Autodesk Inventor part; units mm, degrees
ref_plane "YZ Plane" through (0, 0, 0) normal (1, 0, 0) x (0, 1, 0)
ref_plane "XZ Plane" through (0, 0, 0) normal (0, 1, 0) x (-1, 0, 0)
ref_plane "XY Plane" through (0, 0, 0) normal (0, 0, 1) x (1, 0, 0)
sketch "Sketch1" plane through (0, 0, 0) normal (0, 1, 0) x (-1, 0, 0)
  line L0 (10.3823, 13.6045) -> (-19.4881, 13.6045)
  line L1 (-19.4881, 13.6045) -> (-19.4881, -34.6555)
  line L2 (-19.4881, -34.6555) -> (10.3823, -34.6555)
  line L3 (10.3823, -34.6555) -> (10.3823, 13.6045)
  point P0 (0, 0)
  dimension "d0" = 48.26
  dimension "d1" = 29.8704
extrude "Extrusion1" add sketch "Sketch1" along normal blind 20.193
fillet "Fillet1" radius 3.175 2 edges at (19.4881, 20.193, -10.5255) (-10.3823, 20.193, -10.5255)
sketch "Sketch2" plane through (0, 0, 0) normal (0, -1, 0) x (1, 0, 0)
  line L0 (13.0111, -34.6555) -> (13.0111, -42.2755)
  line L1 (19.4881, 13.6045) -> (19.4881, -34.6555)
  line L2 (13.0111, -42.2755) -> (6.7881, -42.2755)
  line L3 (6.7881, -42.2755) -> (6.7881, -34.6555)
  line L4 (6.7881, -36.6113) -> (2.3177, -36.6113)
  line L5 (2.3177, -34.6555) -> (2.3177, -42.2755)
  line L6 (2.3177, -42.2755) -> (-3.9053, -42.2755)
  line L7 (-3.9053, -42.2755) -> (-3.9053, -34.6555)
  line L8 (-10.3823, -34.6555) -> (-10.3823, 13.6045)
  line L9 (19.4881, -10.5255) -> (-10.3823, -10.5255) construction
  line L10 (13.0111, 13.6045) -> (13.0111, 21.2245)
  line L11 (13.0111, 21.2245) -> (6.7881, 21.2245)
  line L12 (6.7881, 21.2245) -> (6.7881, 13.6045)
  line L13 (6.7881, 15.5603) -> (2.3177, 15.5603)
  line L14 (2.3177, 13.6045) -> (2.3177, 21.2245)
  line L15 (2.3177, 21.2245) -> (-3.9053, 21.2245)
  line L16 (-3.9053, 21.2245) -> (-3.9053, 13.6045)
  line L17 (13.0111, -34.6555) -> (6.7881, -34.6555)
  line L18 (2.3177, -34.6555) -> (-3.9053, -34.6555)
  line L19 (19.4881, -34.6555) -> (-10.3823, -34.6555)
  line L20 (6.7881, -34.6555) -> (2.3177, -34.6555)
  line L21 (13.0111, 13.6045) -> (6.7881, 13.6045)
  line L22 (-10.3823, 13.6045) -> (19.4881, 13.6045)
  line L23 (6.7881, 13.6045) -> (2.3177, 13.6045)
  line L24 (2.1667, 13.6045) -> (-3.9053, 13.6045)
  line L25 (6.7881, 13.6045) -> (2.3177, 13.6045)
  line L26 (2.3177, 13.6045) -> (2.3177, 15.5603)
  line L27 (2.3177, 15.5603) -> (6.7881, 15.5603)
  line L28 (6.7881, 15.5603) -> (6.7881, 13.6045)
  line L29 (6.7881, -36.6113) -> (2.3177, -36.6113)
  line L30 (2.3177, -36.6113) -> (2.3177, -34.6555)
  line L31 (2.3177, -34.6555) -> (6.7881, -34.6555)
  line L32 (6.7881, -34.6555) -> (6.7881, -36.6113)
  line L33 (-3.9053, 13.6045) -> (2.3177, 13.6045)
  line L34 (2.3177, 13.6045) -> (2.3177, 21.2245)
  line L35 (2.3177, 21.2245) -> (-3.9053, 21.2245)
  line L36 (-3.9053, 21.2245) -> (-3.9053, 13.6045)
  point P0 (0, 0)
  dimension "d5" = 6.477
  dimension "d6" = 7.62
  dimension "d7" = 6.223
  dimension "d9" = 4.4704
  dimension "d10" = 6.223
  dimension "d11" = 7.62
  dimension "d12" = 29.8704
  dimension "d13" = 4.4704
  dimension "d15" = 6.477
  dimension "d16" = 6.477
  dimension "d17" = 6.477
extrude "Extrusion2" add sketch "Sketch2" against normal blind 1.8542 contours L0 L2 L3 L17 | L3 L4 L5 L19 | L5 L6 L7 L18 | L21 L12 L11 L10 | L22 L14 L13 L12 | L22 L16 L15 L14
fillet "Fillet2" radius 2.2352 4 edges at (6.7881, 0.9271, 15.5603) (2.3177, 0.9271, 15.5603) (6.7881, 0.9271, -36.6113) (2.3177, 0.9271, -36.6113)
fillet "Fillet3" radius 2.2352 4 edges at (-3.9053, 0.9271, -42.2755) (13.0111, 0.9271, -42.2755) (13.0111, 0.9271, 21.2245) (-3.9053, 0.9271, 21.2245)
sketch "Sketch3" plane through (16.3131, 20.193, -34.6555) normal (0, 0, -1) x (-1, 0, 0)
  circle A0 centre (5.5372, -11.9126) radius 4.2418
  circle A1 centre (17.3736, -11.9126) radius 4.2418
  line L0 (20.2184, -20.193) -> (26.6954, -20.193)
  line L1 (-3.175, -20.193) -> (3.302, -20.193)
  line L2 (-3.175, -20.193) -> (-3.175, -3.175)
  line L3 (26.6954, -20.193) -> (26.6954, -3.175)
  point P0 (16.3131, -20.193)
  dimension "d22" = 8.4836
  dimension "d23" = 8.4836
  dimension "d24" = 8.2804
  dimension "d25" = 8.2804
  dimension "d26" = 11.8364
  dimension "d27" = 4.4704
  dimension "d28" = 5.08
extrude "Extrusion3" add sketch "Sketch3" along normal blind 2.0066 and the other way blind 50.2666
equation "\"d10\" = d7"
equation "\"d11\" = d6"
equation "\"d13\" = d9"
equation "\"d23\" = d22"
equation "\"d25\" = d24"
properties part number "LED Driver"
Here's how the part is built. I have some questions about the finished solid (model axes, mm). A direction names the side the tool comes from. Give positions to 0.01 mm unless a question says otherwise; leave off trailing zeros. Order: outer loops, then holes, each group sorted by start corner. A loop starts at its lowest first (then second) coordinate and runs counter-clockwise, first axis right, second up. Notation, with made-up numbers: M 40,17.25 L 98,17.25 A23 ccw 98,31.25 Z; hole C 73.25,51.25 d9. An arc over 180 degrees is marked long. Use a Markdown table: item, result. Add a question column.
1. Suppose I cut it at D-D (x = -2.75). List the corners of the cut face in (y, z) for me.
2. I need wall thicknesses on probe 1 along X at (y, z) = (8.5, 15); probe 2 along Z at (x, y) = (-7.5, 2.5); probe 3 along X at (y, z) = (9, 14). Which ranges of each line are inside material? Lowest first, please. Write a range as from..to.
3. For pin 1 Ø2.5 at (x, y) = (10.5, 7.5) entering from +Z; pin 2 Ø4 at (x, z) = (5, 17.5) entering from +Y; pin 3 Ø6 at (x, y) = (8.5, 8) entering from -Z, each with a flat end and sliding along its axis, tell me the tip position at first contact or that it passes through.
4. On a 3-axis mill with a long thin cutter (end or side, diameter ignored), from which of +Z, -Z, +X, -X, +Y, -Y can I reach the whole of each face in a straight line? I mean faces 4 (the flat face through (-3.905, 1, -37)), 5 (the cylindrical face through (6.12, 0.94, -37.25)), 6 (the cylindrical face through (14.142, 5.699, 14.594)). Say none if no direction works.
5. Suppose I cut it at B-B (x = 14). List the corners of the cut face in (y, z) for me.
6. Suppose I cut it at C-C (y = 9.5). List the corners of the cut face in (x, z) for me.
7. Suppose I cut it at A-A (y = 6.5). List the corners of the cut face in (x, z) for me.
8. If we mould it in two halves opening along Y, with no side actions, what happens to faces 1 (the flat face through (4, 1.854, 15)), 2 (the flat face through (-1, 8, 15.611)), 3 (the cylindrical face through (-9.428, 19.288, -10.188))? For each: +Y half, -Y half, draft (parallel to the pull), parting line (faces both ways), or undercut.
Results list:
| question | item | result |
|---|---|---|
| 1 | outline | M 0,-42 L 1.85,-42 L 1.85,-34.66 L 4.39,-34.66 L 4.39,-36.66 L 12.17,-36.66 L 12.17,-34.66 L 20.19,-34.66 L 20.19,13.6 L 12.17,13.6 L 12.17,15.61 L 4.39,15.61 L 4.39,13.6 L 1.85,13.6 L 1.85,20.95 L 0,20.95 Z |
| 2 | probe 1 | x = -5.3..3.18, 6.54..15.01 |
| 2 | probe 2 | z = -34.66..13.6 |
| 2 | probe 3 | x = -5.24..3.12, 6.6..14.96 |
| 3 | pin 1 | stops at z = 15.61 |
| 3 | pin 2 | stops at y = 1.85 |
| 3 | pin 3 | stops at z = -36.66 |
| 4 | face 4 | -Z, -X, -Y |
| 4 | face 5 | -Z, +Y, -Y |
| 4 | face 6 | +Z |
| 5 | outline | M 0,-34.66 L 5.52,-34.66 L 5.52,-36.66 L 11.04,-36.66 L 11.04,-34.66 L 20.19,-34.66 L 20.19,13.6 L 11.04,13.6 L 11.04,15.61 L 5.52,15.61 L 5.52,13.6 L 0,13.6 Z |
| 6 | outline | M -10.38,-34.66 L -5.12,-34.66 L -5.12,-36.66 L 3,-36.66 L 3,-34.66 L 6.71,-34.66 L 6.71,-36.66 L 14.84,-36.66 L 14.84,-34.66 L 19.49,-34.66 L 19.49,13.6 L 14.84,13.6 L 14.84,15.61 L 6.71,15.61 L 6.71,13.6 L 3,13.6 L 3,15.61 L -5.12,15.61 L -5.12,13.6 L -10.38,13.6 Z |
| 7 | outline | M -10.38,-34.66 L -4.91,-34.66 L -4.91,-36.66 L 2.79,-36.66 L 2.79,-34.66 L 6.93,-34.66 L 6.93,-36.66 L 14.63,-36.66 L 14.63,-34.66 L 19.49,-34.66 L 19.49,13.6 L 14.63,13.6 L 14.63,15.61 L 6.93,15.61 L 6.93,13.6 L 2.79,13.6 L 2.79,15.61 L -4.91,15.61 L -4.91,13.6 L -10.38,13.6 Z |
| 8 | face 1 | undercut |
| 8 | face 2 | draft |
| 8 | face 3 | +Y half |
